Work out the finished part from the listing and answer in its coordinate system (mm). Round coordinates to 2 decimals unless told otherwise and drop trailing zeros. Order: outer loops, then holes, each group sorted by start corner. A loop starts at its lowest first (then second) coordinate and runs counter-clockwise, first axis right, second up. Notation, with made-up numbers: M 82,54.5 L 135,54.5 A23 cw 135,64.5 Z; hole C 78,-20 d6. An arc over 180 degrees is marked long. Answer as a JSON object with one key per item and string values. Group by question number.
from build123d import *

# Parameters (mm, degrees)
EXTRUDE1_DEPTH      = 4.7625
EXTRUDE1_DEPTH_BACK = 4.7625


with BuildPart() as part:
    # Sketch1 → Extrude1 (new body, two sides)
    with BuildSketch(Plane.XY) as extrude1_sk:
        with BuildLine():
            Line((-0.48777528, -0.086007942), (-0.787944683, -0.138935907))
            ThreePointArc((-0.787944683, -0.138935907), (0.8001, 0), (-0.787944683, 0.138935907))
            Line((-0.787944683, 0.138935907), (-0.48777528, 0.086007942))
            ThreePointArc((-0.48777528, 0.086007942), (0.4953, 0), (-0.48777528, -0.086007942))
        make_face()
    extrude(amount=EXTRUDE1_DEPTH)
    extrude(extrude1_sk.sketch, amount=-EXTRUDE1_DEPTH_BACK)

    # Sketch2 → Cut-Revolve1 (revolve, cut)
    with BuildSketch(Plane(origin=(0, 0, 0), x_dir=(0, 0, -1), z_dir=(1, 0, 0))):
        Polygon((4.7625, 0.73914), (4.2291, 0.8001), (4.7625, 0.8001), align=None)
    cut_revolve1 = revolve(axis=Axis((0, 0, -4.7625), (0, 0, 1)), mode=Mode.SUBTRACT)

    # Mirror1: Cut-Revolve1 across plane
    add(cut_revolve1.mirror(Plane.XY), mode=Mode.SUBTRACT)


solid = part.part
Item 1: Find section A-A (x = 0). Give the vertices of the cut face in (y, z).
Item 2: Find section C-C (z = -2). Give the vertices of the cut face in (x, y).
Item 3: The mould has two halves that part along Y. Classify faces 1 (the cylindrical face through (0.495, 0.021, 0.067)), 2 (the cylindrical face through (0.8, 0, 0.1)): +Y half, -Y half, draft (parallel to the pull), parting line (faces both ways), or undercut.
Item 4: Consider L1, parallel to Y at x = 0, z = -1.5; L2, parallel to X at y = 0.3, z = 0.75; L3, parallel to X at y = 0, z = 1.5. Determine where each line is inside the solid, lowest interval first.
Item 5: Find section B-B (y = 0). Give the vertices of the cut face in (x, z).
Responses:
{
 "1": {"outline": "M -0.8,-4.23 L -0.74,-4.76 L -0.5,-4.76 L -0.5,4.76 L -0.74,4.76 L -0.8,4.23 Z; M 0.5,-4.76 L 0.74,-4.76 L 0.8,-4.23 L 0.8,4.23 L 0.74,4.76 L 0.5,4.76 Z"},
 "2": {"outline": "M -0.79,-0.14 A0.8 ccw long -0.79,0.14 L -0.49,0.09 A0.5 cw long -0.49,-0.09 Z"},
 "3": {"face 1": "undercut", "face 2": "parting line"},
 "4": {"L1": "y = -0.8 to -0.5, 0.5 to 0.8", "L2": "x = -0.74 to -0.39, 0.39 to 0.74", "L3": "x = 0.5 to 0.8"},
 "5": {"outline": "M 0.5,-4.76 L 0.74,-4.76 L 0.8,-4.23 L 0.8,4.23 L 0.74,4.76 L 0.5,4.76 Z"}
}
